Build history of the part. All positions in model axes, mm. A direction names the side the tool comes from. Round coordinates to 2 decimals unless told otherwise and drop trailing zeros. Write each loop counter-clockwise with the first axis right and the second up, starting at its lowest first coordinate (ties: lowest second). Pieces come first, ordered by that corner, then holes. Notation, with made-up numbers: (22.25, -5) -> (55.25, -5) arc R25 ccw to (55.25, 33) -> close; hole circle Ø10 at (-38, 22). An arc over 180 degrees is marked (long way). Return JSON: item names as keys, results as strings.
Autodesk Inventor part; units mm, degrees
ref_plane "YZ Plane" through (0, 0, 0) normal (1, 0, 0) x (0, 1, 0)
ref_plane "XZ Plane" through (0, 0, 0) normal (0, 1, 0) x (-1, 0, 0)
ref_plane "XY Plane" through (0, 0, 0) normal (0, 0, 1) x (1, 0, 0)
sketch "Sketch7" plane through (0, 0, 0) normal (0, 0, 1) x (1, 0, 0)
  circle A0 centre (0, 0) radius 35.5
  dimension "d32" = 71
extrude "Extrusion3" add sketch "Sketch7" along normal blind 60
sketch "Sketch9" plane through (0, 0, 60) normal (0, 0, 1) x (1, 0, 0)
  circle A0 centre (0, 0) radius 34.5
  dimension "d35" = 69
extrude "Extrusion4" cut sketch "Sketch9" against normal blind 58
fillet "Fillet3" radius 1 1 edges at (-35.5, 0, 0)
fillet "Fillet4" radius 1 1 edges at (-35.5, 0, 60)
sketch "Sketch10" plane through (0, 0, 0) normal (0, 0, -1) x (-1, 0, 0)
  circle A0 centre (0, 0) radius 5
  dimension "d40" = 10
hole "Hole4" at (0, 0, 0) direction (0, 0, 1) diameter 10 end through all
properties part number "expo7" material "Glass, Cast, Clear"
Q1. Wall check: L1, parallel to Y at x = -0.5, z = 51; L2, parallel to Y at x = 0, z = 1; L3, parallel to Z at x = -19, y = -25.5. Give the ranges that are in metal, low to high.
Verdict:
{"L1": "y = -35.5 to -34.5, 34.5 to 35.5", "L2": "y = -35.5 to -5, 5 to 35.5", "L3": "z = 0 to 2"}
Q2. 3-axis set-ups, long thin cutter, end or side, ignore diameter. For faces 1 (the cylindrical face through (4.88, -1.08, 1.01)), 2 (the flat face through (0, -7, 2)): which of +Z, -Z, +X, -X, +Y, -Y reach the whole face in a straight line?
Verdict:
{"face 1": "+Z, -Z", "face 2": "+Z"}
Q3. Two-plate mould, pull along Y, no slides. Class faces 3 (the flat face through (0, -7, 0)), 4 (the cylindrical face through (-7.696, 34.656, 29.594)), 5 (the cylindrical face through (32.907, 10.363, 31.406)): +Y half, -Y half, draft (parallel to the pull), parting line (faces both ways), or undercut.
Verdict:
{"face 3": "draft", "face 4": "parting line", "face 5": "undercut"}
Q4. Saw through at C-C on z = 37.5. List the corners of the cut face in (x, y), then the cut area to 3 significant figures.
Verdict:
{"outline": "circle Ø71 at (0, 0); hole circle Ø69 at (0, 0)", "area": "220 mm²"}
Q5. Pin check, flat tips, straight feed: pin 1 Ø4 at (y, z) = (28, 18.5) entering from -X; pin 2 Ø2 at (x, y) = (0, -20.5) entering from +Z; pin 3 Ø1.5 at (y, z) = (-27.5, 9.5) entering from -X. Stop position of each tip, or through.
Verdict:
{"pin 1": "stops at x = -24.17", "pin 2": "stops at z = 2", "pin 3": "stops at x = -23.34"}
